Build history of the part. All positions in model axes, mm. Face numbers are marked on the shaded views. A direction names the side the tool comes from. Coordinates: 2 decimals unless noted, no trailing zeros. Write each loop counter-clockwise with the first axis right and the second up, starting at its lowest first coordinate (ties: lowest second). Pieces come first, ordered by that corner, then holes. Notation, with made-up numbers: (25, -29.75) -> (70, -29.75) arc R17 cw to (70, -9.75) -> close; hole circle Ø10 at (-39.75, -24.5). An arc over 180 degrees is marked (long way). Write each question's results on one line, items separated by ' | '. Start each with the question number.
Q1. Saw through at B-B on x = 0. Give the cut face in (y, z).
Q2. Drop flat-ended pins along their axis: pin 1 Ø8 at (x, z) = (-9, 2) entering from +Y; pin 2 Ø2 at (x, z) = (-15, -13) entering from +Y; pin 3 Ø4 at (x, y) = (-12, 2.5) entering from -Z; pin 4 Ø4 at (x, y) = (11, 4.5) entering from -Z. Give the stop position or say it passes through.
Q3. Drill centre lines: line 1 (X direction, y = 4.5, z = 0); line 2 (X direction, y = 5.75, z = -13.5); line 3 (Z direction, x = 15.5, y = 1.75). Where is each one in solid material? Low to high.
Q4. Two-plate mould, pull along Z, no slides. Class the marked faces 1, 2 and 3: released by +Z, released by -Z, zero draft, split by the parting line, or undercut.
Q5. Tool access for the marked faces 4, 5 and 6: list every direction of +Z, -Z, +X, -X, +Y, -Y with a clear straight run to the whole face (end or side of a thin tool).
Q6. Saw through at C-C on z = 9. Give the cut face in (x, y), and give its area (3 significant figures).
Q7. Saw through at D-D on z = -13. Give the cut face in (x, y), and give its area (3 significant figures).
Q8. Saw through at A-A on z = 0. Give the cut face in (x, y).
from build123d import *

# Parameters (mm, degrees)
SKETCH1_R           = 8
BOSS_EXTRUDE1_DEPTH = 7.5
SKETCH2_W           = 24
SKETCH2_H           = 1
BOSS_EXTRUDE2_DEPTH = 7.5
SKETCH5_W           = 30
SKETCH5_H           = 10
SKETCH6_R           = 20.6375
BOSS_EXTRUDE3_DEPTH = 2
SKETCH7_R           = 4
CUT_EXTRUDE2_DEPTH  = 31.69304176


with BuildPart() as part:
    # Sketch1 → Boss-Extrude1 (new body)
    with BuildSketch(Plane(origin=(0, 0, 0), x_dir=(1, 0, 0), z_dir=(0, 1, 0))):
        with Locations(Location((0, 0, 0), (0, 0, 270))):
            Circle(SKETCH1_R)
    extrude(amount=BOSS_EXTRUDE1_DEPTH)

    # Sketch2 → Boss-Extrude2 (add)
    with BuildSketch(Plane.XZ):
        with Locations((17.4625, 0)):
            Rectangle(SKETCH2_W, SKETCH2_H)
        Polygon((27.514683768, -10.546614783), (4.962060869, -2.338131343), (5.304081013, -1.398438723), (27.856703912, -9.606922162), align=None)
        Polygon((22.248190601, -19.321152172), (3.863123966, -3.894249539), (4.505911575, -3.128205096), (22.89097821, -18.555107729), align=None)
        Polygon((14.298237298, -25.765273459), (2.298237298, -4.980663768), (3.164262702, -4.480663768), (15.164262702, -25.265273459), align=None)
        Polygon((4.623705558, -29.101722512), (0.456149294, -5.46633644), (1.440957047, -5.292688262), (5.608513311, -28.928074334), align=None)
        Polygon((-5.608513311, -28.928074334), (-1.440957047, -5.292688262), (-0.456149294, -5.46633644), (-4.623705558, -29.101722512), align=None)
        Polygon((-15.164262702, -25.265273459), (-3.164262702, -4.480663768), (-2.298237298, -4.980663768), (-14.298237298, -25.765273459), align=None)
        Polygon((-22.89097821, -18.555107729), (-4.505911575, -3.128205096), (-3.863123966, -3.894249539), (-22.248190601, -19.321152172), align=None)
        Polygon((-27.856703912, -9.606922162), (-5.304081013, -1.398438723), (-4.962060869, -2.338131343), (-27.514683768, -10.546614783), align=None)
        with Locations((-17.4625, 0)):
            Rectangle(SKETCH2_W, SKETCH2_H)
        Polygon((-27.514683768, 10.546614783), (-4.962060869, 2.338131343), (-5.304081013, 1.398438723), (-27.856703912, 9.606922162), align=None)
        Polygon((-22.248190601, 19.321152172), (-3.863123966, 3.894249539), (-4.505911575, 3.128205096), (-22.89097821, 18.555107729), align=None)
        Polygon((-14.298237298, 25.765273459), (-2.298237298, 4.980663768), (-3.164262702, 4.480663768), (-15.164262702, 25.265273459), align=None)
        Polygon((-4.623705558, 29.101722512), (-0.456149294, 5.46633644), (-1.440957047, 5.292688262), (-5.608513311, 28.928074334), align=None)
        Polygon((5.608513311, 28.928074334), (1.440957047, 5.292688262), (0.456149294, 5.46633644), (4.623705558, 29.101722512), align=None)
        Polygon((15.164262702, 25.265273459), (3.164262702, 4.480663768), (2.298237298, 4.980663768), (14.298237298, 25.765273459), align=None)
        Polygon((22.89097821, 18.555107729), (4.505911575, 3.128205096), (3.863123966, 3.894249539), (22.248190601, 19.321152172), align=None)
        Polygon((27.856703912, 9.606922162), (5.304081013, 1.398438723), (4.962060869, 2.338131343), (27.514683768, 10.546614783), align=None)
    extrude(amount=-BOSS_EXTRUDE2_DEPTH)

    # Sketch5 → Cut-Revolve1 (revolve, cut)
    with BuildSketch(Plane(origin=(0, 0, 0), x_dir=(0, 0, -1), z_dir=(1, 0, 0))):
        with Locations((32.4625, 4)):
            Rectangle(SKETCH5_W, SKETCH5_H)
    revolve(axis=Axis((0, 0, 0), (0, 1, 0)), mode=Mode.SUBTRACT)

    # Sketch6 → Boss-Extrude3 (add)
    with BuildSketch(Plane(origin=(0, 0, 0), x_dir=(1, 0, 0), z_dir=(0, 1, 0))):
        with Locations(Location((0, 0, 0), (0, 0, 270))):
            Circle(SKETCH6_R)
    extrude(amount=-BOSS_EXTRUDE3_DEPTH)

    # Sketch7 → Cut-Extrude2 (cut, through all)
    with BuildSketch(Plane(origin=(0, 7.5, 0), x_dir=(1, 0, 0), z_dir=(0, 1, 0))):
        with Locations(Location((0, 0, 0), (0, 0, 270))):
            Circle(SKETCH7_R)
    extrude(amount=-CUT_EXTRUDE2_DEPTH, mode=Mode.SUBTRACT)


solid = part.part
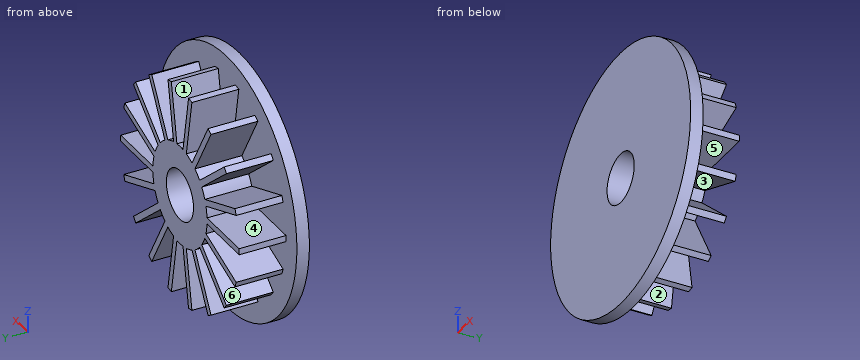
Returned:
1) outline: (-2, -20.64) -> (0, -20.64) -> (0, -8) -> (7.5, -8) -> (7.5, -4) -> (-2, -4) -> close; (-2, 4) -> (7.5, 4) -> (7.5, 8) -> (0, 8) -> (0, 20.64) -> (-2, 20.64) -> close
2) pin 1: stops at y = 7.5 | pin 2: stops at y = 0 | pin 3: stops at z = -11.6 | pin 4: stops at z = -14.96
3) line 1: x = -17.46 to -4, 4 to 17.46 | line 2: x = -8.37 to -7.22, -2.89 to -1.87, 1.87 to 2.89, 7.22 to 8.37 | line 3: z = -6.17 to -5.11, -0.5 to 0.5, 5.11 to 6.17
4) face 1: released by +Z | face 2: released by -Z | face 3: undercut
5) face 4: -X, +Y | face 5: +X, +Y | face 6: +Y
6) outline: (-18.57, -2) -> (18.57, -2) -> (18.57, 0) -> (11.5, 0) -> (11.5, 7.5) -> (9.95, 7.5) -> (9.95, 0) -> (5.77, 0) -> (5.77, 7.5) -> (4.62, 7.5) -> (4.62, 0) -> (2.09, 0) -> (2.09, 7.5) -> (1.08, 7.5) -> (1.08, 0) -> (-1.08, 0) -> (-1.08, 7.5) -> (-2.09, 7.5) -> (-2.09, 0) -> (-4.62, 0) -> (-4.62, 7.5) -> (-5.77, 7.5) -> (-5.77, 0) -> (-9.95, 0) -> (-9.95, 7.5) -> (-11.5, 7.5) -> (-11.5, 0) -> (-18.57, 0) -> close | area: 130 mm2
7) outline: (-16.03, -2) -> (16.03, -2) -> (16.03, 0) -> (8.08, 0) -> (8.08, 7.5) -> (6.93, 7.5) -> (6.93, 0) -> (2.8, 0) -> (2.8, 7.5) -> (1.78, 7.5) -> (1.78, 0) -> (-1.78, 0) -> (-1.78, 7.5) -> (-2.8, 7.5) -> (-2.8, 0) -> (-6.93, 0) -> (-6.93, 7.5) -> (-8.08, 7.5) -> (-8.08, 0) -> (-16.03, 0) -> close | area: 96.7 mm2
8) outline: (-20.64, -2) -> (-4, -2) -> (-4, 7.5) -> (-17.46, 7.5) -> (-17.46, 0) -> (-20.64, 0) -> close; (4, -2) -> (20.64, -2) -> (20.64, 0) -> (17.46, 0) -> (17.46, 7.5) -> (4, 7.5) -> close
